from build123d import *

# Parameters (mm, degrees)
F2_R     = 7
F4_DEPTH = 25
F6_DEPTH = 25


with BuildPart() as f1:
    # F0 (on Right) → F1 (revolve)
    with BuildSketch(Plane.YZ):
        Polygon((-237.755094, 7.5), (-237.755094, 0), (262.244906, 0), (262.244906, 7.5), (237.244906, 7.5), (237.244906, 32), (-212.755094, 32), (-212.755094, 7.5), align=None)
    revolve(axis=Axis((0, 12.244906, 0), (0, -1, 0)))

    # F2
    f2_edges = [f1.edges().sort_by_distance(p)[0] for p in [
        (0, -212.755094, -32),
        (0, 237.244906, -32),
    ]]
    fillet(f2_edges, radius=F2_R)

    # F3 (on face) → F4 (cut, through all)
    with BuildSketch(Plane.XZ.offset(237.755094)):
        Polygon((-0.5, -6), (-7.974903, -6), (-7.77278, -10.850932), (8.599116, -10.850932), (8.599116, -6), (0.5, -6), (0.5, -3.27135), (-0.5, -3.27135), align=None)
    extrude(amount=-F4_DEPTH, mode=Mode.SUBTRACT)

    # F5 (on face) → F6 (cut, through all)
    with BuildSketch(Plane(origin=(0, 262.244906, 0), x_dir=(-1, 0, 0), z_dir=(0, 1, 0))):
        Polygon((9.790156, -10.28766), (8.146554, -6), (0.5, -6), (0.5, -3.27135), (-0.5, -3.27135), (-0.5, -6), (-9.718692, -6), (-10.433301, -10.787886), align=None)
    extrude(amount=-F6_DEPTH, mode=Mode.SUBTRACT)


solid = f1.part
Could you check a few things on this model? Use its own coordinates, in mm. A direction names the side the tool comes from. Coordinates: 2 decimals unless noted, no trailing zeros. Write each loop counter-clockwise with the first axis right and the second up, starting at its lowest first coordinate (ties: lowest second). Pieces come first, ordered by that corner, then holes. Notation, with made-up numbers: (82, -14.75) - (125, -14.75) arc R11 cw to (125, -9.75) - close; hole circle Ø3 at (67.25, 50). An arc over 180 degrees is marked (long way). Put each result on its own line as item: value. Start each with the question number.
Q1. I'm going to push flat-ended pins straight in: P1, Ø6, axis at y = 176, z = -1, coming from the -X side; P2, Ø6, axis at x = -6, z = -17.5, coming from the +Y side; P3, Ø1.1, axis at x = 0, y = -228.5, coming from the -Z side. Where does each tip first touch, or does it pass through?
Q2. I want a section at A-A on y = -153.5. Write out the boundary of the cut face in (x, z), plus the area to 3 significant figures.
Q3. Please list where these lines run through material, in increasing order: L1, parallel to Y at x = 24, z = 6.5; L2, parallel to X at y = 177, z = 2.5; L3, parallel to Z at x = 2, y = 147.
Q4. Which directions (+Z, -Z, +X, -X, +Y, -Y) give clear straight access to the entire face, cutting with the end or side of a thin tool? Please do faces 1 (the cylindrical face through (31.24, 9.19, -6.94)), 2 (the cylindrical face through (0.262, -225.43, 7.495)), 3 (the cylindrical face through (0.262, 249.57, 7.495)).
Checks:
1. P1: x = -32
1. P2: y = 237.24
1. P3: z = -6
2. outline: circle Ø64 at (0, 0)
2. area: 3,220 mm²
3. L1: -212.76 to 237.24
3. L2: -31.9 to 31.9
3. L3: -31.94 to 31.94
4. face 1: +Y, -Y
4. face 2: -Y
4. face 3: +Y
